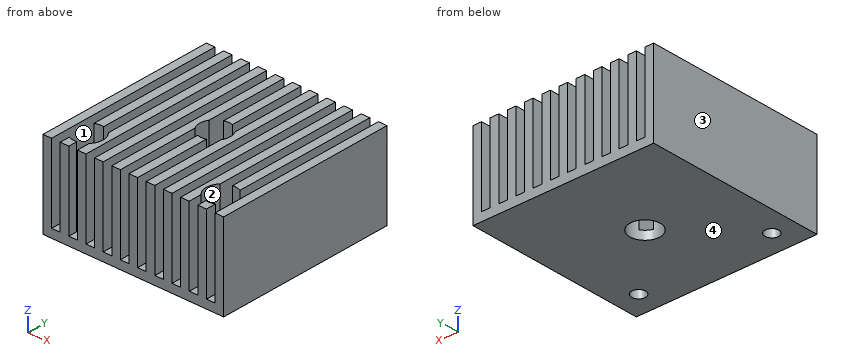
```python
from build123d import *

# Parameters (mm, degrees)
SKETCH1_W               = 42
SKETCH1_H               = 42
BOSS_EXTRUDE1_DEPTH     = 20
CUT_EXTRUDE6_DEPTH      = 63.673758464
CUT_EXTRUDE6_DEPTH_BACK = 42
SKETCH7_W               = 2
SKETCH7_H               = 18
SKETCH8_R               = 1.6
SKETCH8_R_2             = 3.5
CUT_EXTRUDE7_DEPTH      = 2
CUT_EXTRUDE8_START      = -18
SKETCH10_R              = 3.5
CUT_EXTRUDE8_DEPTH      = 18


with BuildPart() as part:
    # Sketch1 → Boss-Extrude1 (new body)
    with BuildSketch(Plane.XY):
        with Locations((21, 21)):
            Rectangle(SKETCH1_W, SKETCH1_H)
    extrude(amount=BOSS_EXTRUDE1_DEPTH)

    # Sketch7 → Cut-Extrude6 (cut, two sides: drawn at the far end of the back side and taken through both)
    with BuildSketch(Plane(origin=(0, 42, 0), x_dir=(1, 0, 0), z_dir=(0, 1, 0)).offset(-CUT_EXTRUDE6_DEPTH_BACK)):
        with Locations((39, -11)):
            Rectangle(SKETCH7_W, SKETCH7_H)
        with Locations((35, -11)):
            Rectangle(SKETCH7_W, SKETCH7_H)
        with Locations((3, -11)):
            Rectangle(SKETCH7_W, SKETCH7_H)
        with Locations((31, -11)):
            Rectangle(SKETCH7_W, SKETCH7_H)
        with Locations((7, -11)):
            Rectangle(SKETCH7_W, SKETCH7_H)
        with Locations((27, -11)):
            Rectangle(SKETCH7_W, SKETCH7_H)
        with Locations((11, -11)):
            Rectangle(SKETCH7_W, SKETCH7_H)
        with Locations((23, -11)):
            Rectangle(SKETCH7_W, SKETCH7_H)
        with Locations((15, -11)):
            Rectangle(SKETCH7_W, SKETCH7_H)
        with Locations((19, -11)):
            Rectangle(SKETCH7_W, SKETCH7_H)
    extrude(amount=CUT_EXTRUDE6_DEPTH + CUT_EXTRUDE6_DEPTH_BACK, mode=Mode.SUBTRACT)

    # Sketch8 → Cut-Extrude7 (cut)
    with BuildSketch(Plane(origin=(0, 0, 0), x_dir=(-1, 0, 0), z_dir=(0, 0, -1))):
        with Locations((-36.5, 5.5)):
            Circle(SKETCH8_R)
        with Locations(Location((-5.5, 5.5, 0), (0, 0, 20.364134806))):
            Circle(SKETCH8_R)
        with Locations((-21, 21)):
            Circle(SKETCH8_R_2)
    extrude(amount=-CUT_EXTRUDE7_DEPTH, mode=Mode.SUBTRACT)

    # Sketch10 → Cut-Extrude8 (cut)
    with BuildSketch(Plane.XY.offset(20).offset(CUT_EXTRUDE8_START)):
        with Locations((36.5, 5.5)):
            Circle(SKETCH10_R)
        with Locations((5.5, 5.5)):
            Circle(SKETCH10_R)
        with Locations(Location((21, 21, 0), (0, 0, 180))):
            Circle(SKETCH10_R)
    extrude(amount=CUT_EXTRUDE8_DEPTH, mode=Mode.SUBTRACT)


solid = part.part
```
Check sheet for the modelled part. Datum: model origin and axes. Units: mm. Face numbers are marked on the shaded views. Coordinates: 2 decimals unless noted, no trailing zeros. Loops run counter-clockwise (first coordinate to the right, second up) from the corner with the lowest first, then second, coordinate; pieces in that order, holes last. Notation, with made-up numbers: M -5,66.5 L -1,66.5 A13 ccw -1,90.5 Z; hole C 56.5,11 d10. An arc over 180 degrees is marked long. Answer as a JSON object with one key per item and string values.
1. Sectioned sample at B-B on y = 5.5. Count the separate pieces of the cut face and the enclosed holes in it, and give its area (3 significant figures).
Outcome:
{"separate pieces": "3", "enclosed holes": "0", "area": "359 mm²"}
2. Release check for a two-part mould opening along X. For the marked faces 1, 2, 3 and 4 record: pulls with the +X half, pulls with the -X half, needs draft (parallel to the pull), parting line crosses it, or undercut.
Outcome:
{"face 1": "undercut", "face 2": "undercut", "face 3": "pulls with the -X half", "face 4": "needs draft"}
3. Sectioned sample at A-A on x = 23. Record the cut outline in (y, z).
Outcome:
{"outline": "M 0,0 L 18.13,0 L 18.13,2 L 0,2 Z; M 23.87,0 L 42,0 L 42,2 L 23.87,2 Z"}
4. Depth check by flat-ended pin: P1, Ø5, axis at x = 23.5, z = 9.5, coming from the -Y side; P2, Ø0.6, axis at x = 19, y = 31.5, coming from the +Z side. Enter the tip coordinate at first touch or a pass-through.
Outcome:
{"P1": "y = 0", "P2": "z = 2"}
5. Scan lines: L1, parallel to Y at x = 5, z = 5.5; L2, parallel to Y at x = 21, z = 8; L3, parallel to Z at x = 6.5, y = 31. Record each from-to range of solid material in increasing order. Write a range as from..to.
Outcome:
{"L1": "0..2.04, 8.96..42", "L2": "0..17.5, 24.5..42", "L3": "0..2"}
